Build history of the part. All positions in model axes, mm. A direction names the side the tool comes from. Coordinates: 2 decimals unless noted, no trailing zeros. Write each loop counter-clockwise with the first axis right and the second up, starting at its lowest first coordinate (ties: lowest second). Pieces come first, ordered by that corner, then holes. Notation, with made-up numbers: M -6.5,-13 L 49.5,-13 A3 cw 49.5,-9 Z; hole C -31,-24 d1. An arc over 180 degrees is marked long. Use CSV: the item, a comma, the result in double quotes. Start each with the question number.
```python
from build123d import *

# Parameters (mm, degrees)
F1_DEPTH = 209.55
F3_DEPTH = 0.4064


# Not quite as in the source:
# - the dataset's text gives a spline's control points without its knots; the knots are read off the source's solid


with BuildPart() as f1:
    # F0 (on Right) → F1 (new body, symmetric)
    with BuildSketch(Plane.YZ):
        Polygon((-139.7, 0), (0, 0), (0, 88.9), (-139.2936, 88.9), (-139.2936, 89.154), (-40.6298144724, 187.8177855276), (-40.9171826682, 188.1051537235), (-139.7, 89.3223363917), align=None)
    extrude(amount=F1_DEPTH, both=True)

    # F2 (on face) → F3 (cut, through all)
    with BuildSketch(Plane(origin=(0, -114.5111681959, 114.5111681959), x_dir=(1, 0, 0), z_dir=(0, -0.7071067812, 0.7071067812))):
        with BuildLine():
            add(Edge.make_bspline(
                [(-30.4346554714, 12.4755289708), (-28.8919356714, 10.9324789708), (-26.7232582714, 10.0343349708), (-24.5415760714, 10.0343349708)],
                knots=[3, 3, 3, 3, 4, 4, 4, 4], degree=3))
            Line((-24.5415760714, 10.0343349708), (-14.2228260714, 10.0343349708))
            add(Edge.make_bspline(
                [(-14.2228260714, 10.0343349708), (-12.0402548714, 10.0343349708), (-9.8723140714, 10.9324789708), (-8.3296196714, 12.4755289708)],
                knots=[0, 0, 0, 0, 1, 1, 1, 1], degree=3))
            add(Edge.make_bspline(
                [(-8.3296196714, 12.4755289708), (-6.7864680714, 14.0182741708), (-5.8884256714, 16.1866213708), (-5.8884256714, 18.3687099708), (-5.8884256714, 20.5508747708), (-6.7864680714, 22.7191711708), (-8.3296196714, 24.2622719708)],
                knots=[1, 1, 1, 1, 2, 2, 2, 3, 3, 3, 3], degree=3))
            add(Edge.make_bspline(
                [(-8.3296196714, 24.2622719708), (-9.8723140714, 25.8049663708), (-12.0402548714, 26.7030849708), (-14.2228260714, 26.7030849708)],
                knots=[3, 3, 3, 3, 4, 4, 4, 4], degree=3))
            Line((-14.2228260714, 26.7030849708), (-24.5415760714, 26.7030849708))
            add(Edge.make_bspline(
                [(-24.5415760714, 26.7030849708), (-26.7232582714, 26.7030849708), (-28.8919356714, 25.8049663708), (-30.4346554714, 24.2622719708)],
                knots=[0, 0, 0, 0, 1, 1, 1, 1], degree=3))
            add(Edge.make_bspline(
                [(-30.4346554714, 24.2622719708), (-31.9773752714, 22.7191711708), (-32.8759510714, 20.5508747708), (-32.8759510714, 18.3687099708), (-32.8759510714, 16.1866213708), (-31.9773752714, 14.0182741708), (-30.4346554714, 12.4755289708)],
                knots=[1, 1, 1, 1, 2, 2, 2, 3, 3, 3, 3], degree=3))
        make_face()
        with BuildLine():
            add(Edge.make_bspline(
                [(50.9739701286, 35.1022299708), (48.2554589286, 37.8204363708), (44.4345115286, 39.4030849708), (40.5900437286, 39.4030849708)],
                knots=[7, 7, 7, 7, 8, 8, 8, 8], degree=3))
            add(Edge.make_bspline(
                [(40.5900437286, 39.4030849708), (36.7460839286, 39.4030849708), (32.9251365286, 37.8204363708), (30.2066253286, 35.1022299708)],
                knots=[0, 0, 0, 0, 1, 1, 1, 1], degree=3))
            add(Edge.make_bspline(
                [(30.2066253286, 35.1022299708), (27.4884189286, 32.3837441708), (25.9056687286, 28.5627713708), (25.9056687286, 24.7187099708), (25.9056687286, 20.8743691708), (27.4884189286, 17.0535741708), (30.2066253286, 14.3355455708)],
                knots=[1, 1, 1, 1, 2, 2, 2, 3, 3, 3, 3], degree=3))
            add(Edge.make_bspline(
                [(30.2066253286, 14.3355455708), (32.9251365286, 11.6170089708), (36.7460839286, 10.0343349708), (40.5900437286, 10.0343349708), (44.4345115286, 10.0343349708), (48.2554589286, 11.6170089708), (50.9739701286, 14.3355455708)],
                knots=[3, 3, 3, 3, 4, 4, 4, 5, 5, 5, 5], degree=3))
            add(Edge.make_bspline(
                [(50.9739701286, 14.3355455708), (53.6921765286, 17.0535741708), (55.2744187286, 20.8743691708), (55.2744187286, 24.7187099708), (55.2744187286, 28.5627713708), (53.6921765286, 32.3837441708), (50.9739701286, 35.1022299708)],
                knots=[5, 5, 5, 5, 6, 6, 6, 7, 7, 7, 7], degree=3))
        make_face()
        with BuildLine():
            add(Edge.make_bspline(
                [(110.7016129286, 45.2649223708), (106.8809957286, 49.0851839708), (101.5114865286, 51.3095127708), (96.1084493286, 51.3095127708)],
                knots=[7, 7, 7, 7, 8, 8, 8, 8], degree=3))
            add(Edge.make_bspline(
                [(96.1084493286, 51.3095127708), (90.7062757286, 51.3095127708), (85.3364109286, 49.0851839708), (81.5161493286, 45.2649223708)],
                knots=[0, 0, 0, 0, 1, 1, 1, 1], degree=3))
            add(Edge.make_bspline(
                [(81.5161493286, 45.2649223708), (77.6955067286, 41.4443305708), (75.4709493286, 36.0747705708), (75.4709493286, 30.6720127708), (75.4709493286, 25.2692549708), (77.6955067286, 19.8992123708), (81.5161493286, 16.0789507708)],
                knots=[1, 1, 1, 1, 2, 2, 2, 3, 3, 3, 3], degree=3))
            add(Edge.make_bspline(
                [(81.5161493286, 16.0789507708), (85.3364109286, 12.2585113708), (90.7062757286, 10.0345127708), (96.1084493286, 10.0345127708), (101.5114865286, 10.0345127708), (106.8809957286, 12.2585113708), (110.7016129286, 16.0789507708)],
                knots=[3, 3, 3, 3, 4, 4, 4, 5, 5, 5, 5], degree=3))
            add(Edge.make_bspline(
                [(110.7016129286, 16.0789507708), (114.5218745286, 19.8992123708), (116.7459493286, 25.2692549708), (116.7459493286, 30.6720127708), (116.7459493286, 36.0747705708), (114.5218745286, 41.4443305708), (110.7016129286, 45.2649223708)],
                knots=[5, 5, 5, 5, 6, 6, 6, 7, 7, 7, 7], degree=3))
        make_face()
        with BuildLine():
            add(Edge.make_bspline(
                [(174.3060069286, 45.9422641708), (170.4119075286, 49.8362111708), (164.9391219286, 52.1032627708), (159.4321479286, 52.1032627708)],
                knots=[7, 7, 7, 7, 8, 8, 8, 8], degree=3))
            add(Edge.make_bspline(
                [(159.4321479286, 52.1032627708), (153.9258597286, 52.1032627708), (148.4526169286, 49.8362111708), (144.5589747286, 45.9422641708)],
                knots=[0, 0, 0, 0, 1, 1, 1, 1], degree=3))
            add(Edge.make_bspline(
                [(144.5589747286, 45.9422641708), (140.6649769286, 42.0482663708), (138.3976713286, 36.5757347708), (138.3976713286, 31.0688877708), (138.3976713286, 25.5620661708), (140.6649769286, 20.0890519708), (144.5589747286, 16.1950541708), (148.4526169286, 12.3014119708), (153.9258597286, 10.0345127708), (159.4321479286, 10.0345127708), (164.9391219286, 10.0345127708), (170.4119075286, 12.3014119708), (174.3060069286, 16.1950541708)],
                knots=[1, 1, 1, 1, 2, 2, 2, 3, 3, 3, 4, 4, 4, 5, 5, 5, 5], degree=3))
            add(Edge.make_bspline(
                [(174.3060069286, 16.1950541708), (178.1996491286, 20.0890519708), (180.4665229286, 25.5620661708), (180.4665229286, 31.0688877708), (180.4665229286, 36.5757347708), (178.1996491286, 42.0482663708), (174.3060069286, 45.9422641708)],
                knots=[5, 5, 5, 5, 6, 6, 6, 7, 7, 7, 7], degree=3))
        make_face()
    extrude(amount=-F3_DEPTH, mode=Mode.SUBTRACT)


solid = f1.part
```
1. Slice it at A-A (y = -57.5). List the corners of the cut face in (x, z), and give its area (3 significant figures).
2. Flat gauge pins, fed straight in: pin 1 (12 mm diameter, centred on x = 93.5, y = -66.5, fed in from +Z); pin 2 (4 mm diameter, centred on x = -83.5, y = -81.5, fed in from +Z); pin 3 (10 mm diameter, centred on x = 103.5, z = 103.5, fed in from -Y). Where does each tip first touch, or does it go through?
3. Slice it at B-B (x = -134). List the corners of the cut face in (y, z), and give its area (3 significant figures).
4. 3-axis set-ups, long thin cutter, end or side, ignore diameter. For faces 1 (the flat face through (3, -69, 88.9)), 2 (the flat face through (-209.55, -71, 54)): which of +Z, -Z, +X, -X, +Y, -Y reach the whole face in a straight line?
5. Drill centre lines: line 1 along Z through (x, y) = (-18.5, -31); line 2 along Z through (x, y) = (-188, -107.5); line 3 along Z through (x, y) = (-181, -53.5). Where is each one in solid material? Low to high. Write a range as from..to.
6. Slice it at C-C (y = -21). List the corners of the cut face in (x, z).
7. Slice it at D-D (z = 95.5). List the corners of the cut face in (x, y), and give its area (3 significant figures).
Established:
1,outline,"M -209.55,0 L 209.55,0 L 209.55,88.9 L -209.55,88.9 Z; M -209.55,170.95 L 209.55,170.95 L 209.55,171.52 L -209.55,171.52 Z"
1,area,"37,500 mm2"
2,pin 1,"stops at z = 168.52"
2,pin 2,"stops at z = 149.52"
2,pin 3,"stops at y = -130.52"
3,outline,"M -139.7,0 L 0,0 L 0,88.9 L -139.29,88.9 L -139.29,89.15 L -40.63,187.82 L -40.92,188.11 L -139.7,89.32 Z"
3,area,"12,500 mm2"
4,face 1,"+X, -X, +Y"
4,face 2,"+Z, -Z, -X, +Y, -Y"
5,line 1,"z = 0..88.9"
5,line 2,"z = 0..88.9, 120.95..121.52"
5,line 3,"z = 0..88.9, 174.95..175.52"
6,outline,"M -209.55,0 L 209.55,0 L 209.55,88.9 L -209.55,88.9 Z"
7,outline,"M -209.55,-133.52 L 209.55,-133.52 L 209.55,-132.95 L -209.55,-132.95 Z"
7,area,"241 mm2"
